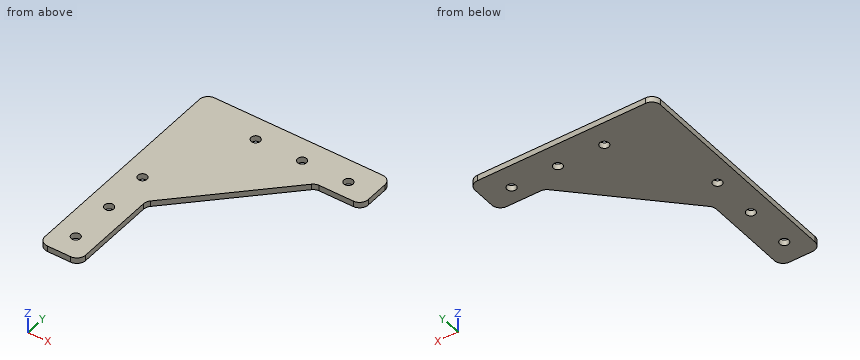
```python
from build123d import *

# Parameters (mm, degrees)
SKETCH1_R           = 2.4892
BOSS_EXTRUDE1_DEPTH = 1.5875
FILLET1_R           = 4.7625


with BuildPart() as part:
    # Sketch1 → Boss-Extrude1 (new, symmetric)
    with BuildSketch(Plane.XY):
        Polygon((0, 0), (0, 127), (101.6, 127), (101.6, 104.775), (76.2, 104.775), (22.225, 50.8), (22.225, 0), align=None)
        with Locations((11.1125, 63.5)):
            Circle(SKETCH1_R, mode=Mode.SUBTRACT)
        with Locations((11.1125, 38.1)):
            Circle(SKETCH1_R, mode=Mode.SUBTRACT)
        with Locations((11.1125, 12.7)):
            Circle(SKETCH1_R, mode=Mode.SUBTRACT)
        with Locations((87.3125, 114.3)):
            Circle(SKETCH1_R, mode=Mode.SUBTRACT)
        with Locations((61.9125, 114.3)):
            Circle(SKETCH1_R, mode=Mode.SUBTRACT)
        with Locations((36.5125, 114.3)):
            Circle(SKETCH1_R, mode=Mode.SUBTRACT)
    extrude(amount=BOSS_EXTRUDE1_DEPTH, both=True)

    # Fillet1
    fillet1_edges = [part.edges().sort_by_distance(p)[0] for p in [
        (22.225, 0, 0),
        (22.225, 50.8, 0),
        (76.2, 104.775, 0),
        (101.6, 104.775, 0),
        (101.6, 127, 0),
        (0, 127, 0),
        (0, 0, 0),
    ]]
    fillet(fillet1_edges, radius=FILLET1_R)


solid = part.part
```
Geometry: final body of the model. Coordinates: model frame, mm. Round coordinates to 2 decimals unless told otherwise and drop trailing zeros. Write each loop counter-clockwise with the first axis right and the second up, starting at its lowest first coordinate (ties: lowest second). Pieces come first, ordered by that corner, then holes.
Item 1: Material intervals for L1, parallel to X at y = 114, z = 0.2; L2, parallel to Y at x = 9.5, z = 1; L3, parallel to Y at x = 92, z = -0.7 (3 decimals), sorted ascending.
Item 2: Section query B-B (y = 38.1). Return loops of the section in (x, z) (1 decimal).
Item 3: Section query D-D (x = 92). Return loops of the section in (y, z) (1 decimal), plus the area to 3 significant figures.
Item 4: Section query A-A (z = -1.05). Return loops of the section in (x, y) (1 decimal).
Item 5: Section query C-C (x = 37). Return loops of the section in (y, z) (1 decimal), plus the area to 3 significant figures.
Item 6: Pin query (flat end, axial travel): P1, Ø3, axis at x = 11.11, y = 12.7, coming from the +Z side; P2, Ø1.6, axis at y = 26.5, z = -0.5, coming from the +X side (3 decimals). Return the tip coordinate at first contact, or that it passes through.
Completed:
1. L1: x = 0 to 34.04, 38.98 to 59.44, 64.38 to 84.84, 89.78 to 101.6
1. L2: y = 0 to 10.8, 14.6 to 36.2, 40 to 61.6, 65.4 to 127
1. L3: y = 104.775 to 127
2. outline: (0, -1.6) - (8.6, -1.6) - (8.6, 1.6) - (0, 1.6) - close; (13.6, -1.6) - (22.2, -1.6) - (22.2, 1.6) - (13.6, 1.6) - close
3. outline: (104.8, -1.6) - (127, -1.6) - (127, 1.6) - (104.8, 1.6) - close
3. area: 70.6 mm2
4. outline: (0, 4.8) arc R4.8 ccw to (4.8, 0) - (17.5, 0) arc R4.8 ccw to (22.2, 4.8) - (22.2, 48.8) arc R4.8 cw to (23.6, 52.2) - (74.8, 103.4) arc R4.8 cw to (78.2, 104.8) - (96.8, 104.8) arc R4.8 ccw to (101.6, 109.5) - (101.6, 122.2) arc R4.8 ccw to (96.8, 127) - (4.8, 127) arc R4.8 ccw to (0, 122.2) - close; hole circle Ø5 at (11.1, 12.7); hole circle Ø5 at (11.1, 38.1); hole circle Ø5 at (11.1, 63.5); hole circle Ø5 at (36.5, 114.3); hole circle Ø5 at (61.9, 114.3); hole circle Ø5 at (87.3, 114.3)
5. outline: (65.6, -1.6) - (111.9, -1.6) - (111.9, 1.6) - (65.6, 1.6) - close; (116.7, -1.6) - (127, -1.6) - (127, 1.6) - (116.7, 1.6) - close
5. area: 180 mm2
6. P1: passes through
6. P2: stops at x = 22.225
